Drawing for the job (mm, zero at the part's lowest x, y, z). Coordinates: 2 decimals unless noted, no trailing zeros. Loops run counter-clockwise (first coordinate to the right, second up) from the corner with the lowest first, then second, coordinate; pieces in that order, holes last. Notation, with made-up numbers: (22, -20) - (37, -20) arc R32 cw to (37, 7) - close; hole circle Ø10 at (73.25, 18.25). An arc over 180 degrees is marked (long way). One line per item, written item: value.
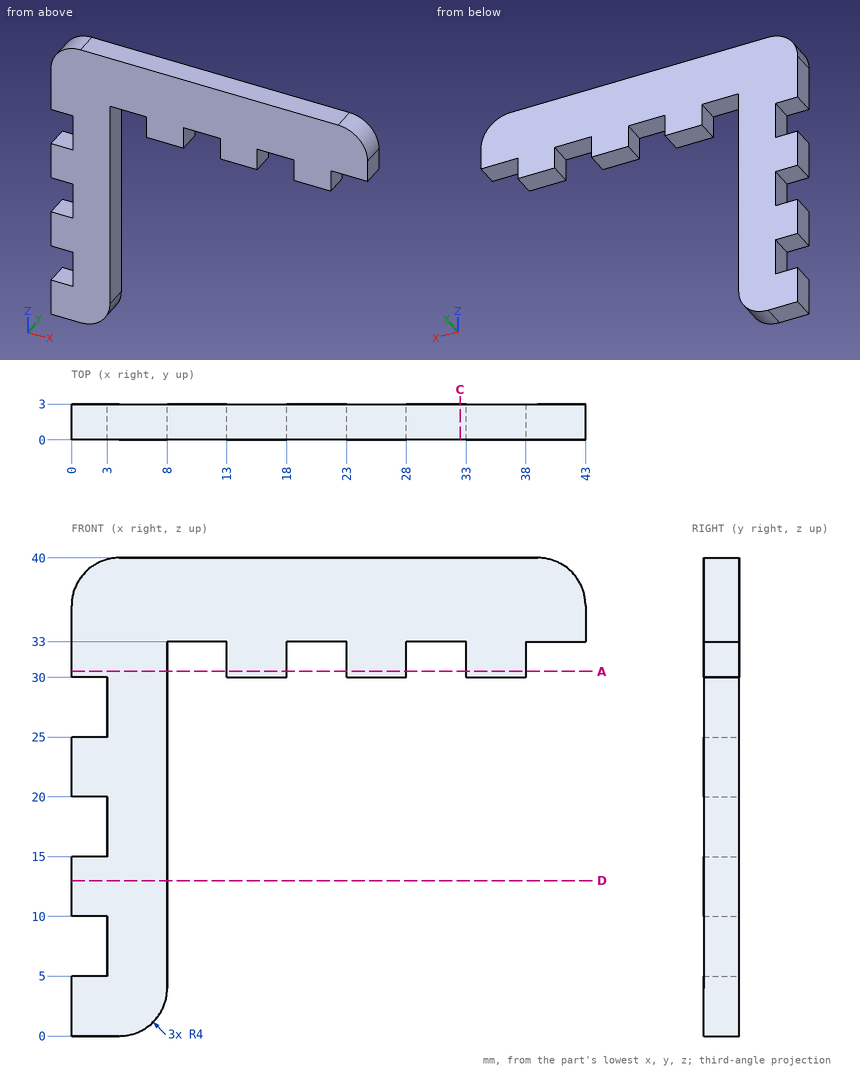
Item 1: Cut at D-D, the plane z = 13. Write the cut outline in (x, y), then the cut area to 3 significant figures.
Check result:
outline: (0, 0) - (8, 0) - (8, 3) - (0, 3) - close
area: 24.0 mm^2
Item 2: Cut at C-C, the plane x = 32.5. Write the cut outline in (y, z).
Check result:
outline: (0, 33) - (3, 33) - (3, 40) - (0, 40) - close
Item 3: Probe probe 1 along X at (y, z) = (0.2, 24.5); probe 2 along Z at (x, y) = (31, 1.75); probe 3 along X at (y, z) = (2.75, 15.5). List the from-to ranges inside material, lowest first. Write a range as from..to.
Check result:
probe 1: x = 0..8
probe 2: z = 33..40
probe 3: x = 3..8
Item 4: Cut at A-A, the plane z = 30.5. Write the cut outline in (x, y).
Check result:
outline: (0, 0) - (8, 0) - (8, 3) - (0, 3) - close; (13, 0) - (18, 0) - (18, 3) - (13, 3) - close; (23, 0) - (28, 0) - (28, 3) - (23, 3) - close; (33, 0) - (38, 0) - (38, 3) - (33, 3) - close
Item 5: Drop flat-ended pins along their axis: P1, Ø0.9, axis at y = 1, z = 27, coming from the -X side; P2, Ø1.5, axis at x = 1, y = 1, coming from the +Z side; P3, Ø0.9, axis at x = 29.5, y = 2, coming from the -Z side. Give the stop position or say it passes through.
Check result:
P1: stops at x = 3
P2: stops at z = 39.31
P3: stops at z = 33
